Here's how the part is built. I have some questions about the finished solid (model axes, mm). A direction names the side the tool comes from. Coordinates: 2 decimals unless noted, no trailing zeros. Write each loop counter-clockwise with the first axis right and the second up, starting at its lowest first coordinate (ties: lowest second). Pieces come first, ordered by that corner, then holes.
Item 1: If we section it at B-B (x = 84.5): Please give me the cut outline in (y, z).
Item 2: For faces 1 (the face through (-2, -150, 1266)), 2 (the face through (-148.99, -80.51, 1266.5)), 3 (the face through (7.81, 140.14, 1479.49)), 4 (the face through (2, 150, 1322)), 5 (the face through (175, 69, 1266)), which set-ups out of +Z, -Z, +X, -X, +Y, -Y let a thin tool reach every point of the face, with its end or its side?
Item 3: If I drill on line 1 (Z direction, x = 0, y = 145.25); line 2 (Z direction, x = 28, y = 63); line 3 (X direction, y = 59.5, z = 1041.5), over which ranges is the centre line in solid material (lowest first)?
Item 4: I'm going to push flat-ended pins straight in: pin 1 Ø5 at (x, z) = (29, 515) entering from +Y; pin 2 Ø12 at (x, z) = (-29, 688) entering from +Y; pin 3 Ø4 at (x, y) = (57.5, 174) entering from +Z; pin 4 Ø1 at (y, z) = (86, 1321) entering from +X. Where does each tip first touch, or does it pass through?
Item 5: If we section it at A-A (z = 1420): Please give me the cut outline in (x, y), then the cut area to 3 significant figures.
Item 6: If we section it at C-C (y = -40): Please give me the cut outline in (x, z).
Item 7: We'd pull the mould along Z, two halves only. Please class faces 6 (the face through (148.99, -80.51, 1266.5)), 7 (the face through (16.273, 140.14, 1303.936)), 8 (the face through (-23.846, 7.509, 513)), 9 (the face through (-3, 4, 0)): +Z half, -Z half, draft (parallel to the pull), parting line (faces both ways), or undercut.
Item 8: If we section it at D-D (z = 1180): Please give me the cut outline in (x, y), then the cut area to 3 significant figures.
Autodesk Fusion 360 part; units mm, degrees
sketch "Schizzo1" plane through (0, 0, 0) normal (0, 0, 1) x (1, 0, 0)
  circle A0 centre (0, 0) radius 250
  dimension "d1" = 500
extrude "Estrusione1" add sketch "Schizzo1" along normal blind 20
sketch "Schizzo2" plane through (0, 0, 20) normal (0, 0, 1) x (-1, 0, 0)
  circle A0 centre (0, 0) radius 250
  circle A1 centre (0, 0) radius 25
  dimension "d4" = 50
extrude "Estrusione2" add sketch "Schizzo2" along normal blind 1000 contours A1
sketch "Schizzo3" plane through (0, 0, 1020) normal (0, 0, 1) x (-1, 0, 0)
  circle A0 centre (0, 0) radius 25
  line L0 (-175, -150) -> (175, -150)
  line L1 (175, -150) -> (175, 150)
  line L2 (175, 150) -> (-175, 150)
  line L3 (-175, 150) -> (-175, -150)
  line L4 (-175, -150) -> (175, 150) construction
  line L5 (175, -150) -> (-175, 150) construction
  line L6 (-123.697, 150) -> (-175, 9.0461)
  line L7 (123.697, 150) -> (175, 9.0461)
  dimension "d7" = 350
  dimension "d8" = 300
  dimension "d11" = 150
  dimension "d12" = 20
  dimension "d13" = 20
extrude "Estrusione3" add sketch "Schizzo3" along normal blind 500 contours A0 | L0 L1 L2 L3 L6 L7
sketch "Schizzo4" plane through (0, 150, 0) normal (0, 1, 0) x (-1, 0, 0)
  line L0 (-175, 1020) -> (175, 1020)
  line L1 (175, 1020) -> (175, 1520)
  line L2 (175, 1520) -> (-175, 1520)
  line L3 (-175, 1520) -> (-175, 1020)
  line L4 (0, 1520) -> (0, 1020) construction
  circle A0 centre (0, 1420) radius 60
  circle A1 centre (0, 1180) radius 125
  dimension "d14" = 120
  dimension "d15" = 250
  dimension "d16" = 100
  dimension "d17" = 160
extrude "Estrusione4" cut sketch "Schizzo4" against normal blind 20 contours A0 | A1
component "Component" placed x (1, 0, 0) y (0, 1, 0) z (0, 0, 1) at (0, 0, 0)
Answer list:
1. outline: (-235.29, 0) - (235.29, 0) - (235.29, 20) - (-235.29, 20) - close; (-150, 1020) - (150, 1020) - (150, 1087.89) - (130, 1087.89) - (130, 1272.11) - (150, 1272.11) - (150, 1520) - (-150, 1520) - close
2. face 1: +Z, +X, -X, -Y
2. face 2: +Z, -X, -Y
2. face 3: +Y
2. face 4: +Z, +X, -X, +Y
2. face 5: +Z, +X, +Y, -Y
3. line 1: z = 0 to 20, 1020 to 1055, 1305 to 1360, 1480 to 1520
3. line 2: z = 0 to 20, 1020 to 1520
3. line 3: x = -175 to 175
4. pin 1: passes through
4. pin 2: stops at y = 9.8
4. pin 3: stops at z = 20
4. pin 4: stops at x = 175
5. outline: (-175, -9.05) - (-123.7, -150) - (123.7, -150) - (175, -9.05) - (175, 150) - (60, 150) - (60, 130) - (-60, 130) - (-60, 150) - (-175, 150) - close
5. area: 95,400 mm2
6. outline: (-246.78, 0) - (246.78, 0) - (246.78, 20) - (-246.78, 20) - close; (-163.73, 1020) - (163.73, 1020) - (163.73, 1520) - (-163.73, 1520) - close
7. face 6: draft
7. face 7: undercut
7. face 8: undercut
7. face 9: -Z half
8. outline: (-175, -9.05) - (-123.7, -150) - (123.7, -150) - (175, -9.05) - (175, 150) - (125, 150) - (125, 130) - (-125, 130) - (-125, 150) - (-175, 150) - close
8. area: 92,800 mm2
